```python
from build123d import *

# Parameters (mm, degrees)
SKETCH1_R           = 10
BOSS_EXTRUDE1_DEPTH = 80
FILLET1_R           = 10
BOSS_EXTRUDE2_START = 64
SKETCH2_R           = 12
SKETCH2_R_2         = 10
BOSS_EXTRUDE2_DEPTH = 6


with BuildPart() as part:
    # Sketch1 → Boss-Extrude1 (new body)
    with BuildSketch(Plane.XY):
        Circle(SKETCH1_R)
    extrude(amount=BOSS_EXTRUDE1_DEPTH)

    # Fillet1
    fillet1_edges = [part.edges().sort_by_distance(p)[0] for p in [
        (-10, 0, 80),
    ]]
    fillet(fillet1_edges, radius=FILLET1_R)

    # Sketch2 → Boss-Extrude2 (add)
    with BuildSketch(Plane.XY.offset(BOSS_EXTRUDE2_START)):
        Circle(SKETCH2_R)
        Circle(SKETCH2_R_2, mode=Mode.SUBTRACT)
    extrude(amount=BOSS_EXTRUDE2_DEPTH)


solid = part.part
```
Build history of the part. All positions in model axes, mm. A direction names the side the tool comes from. Give positions to 0.01 mm unless a question says otherwise; leave off trailing zeros. Loops run counter-clockwise (first coordinate to the right, second up) from the corner with the lowest first, then second, coordinate; pieces in that order, holes last.
Item 1: Drill centre lines: line 1 (X direction, y = 0.5, z = 51.5); line 2 (Y direction, x = 0, z = 61); line 3 (Z direction, x = 3.75, y = 10.5). Where is each one in solid material? Low to high.
Answers follow:
line 1: x = -9.99 to 9.99
line 2: y = -10 to 10
line 3: z = 64 to 70
Item 2: Slice it at A-A, the plane x = 0. List the corners of the cut face in (y, z), and give its area (3 significant figures).
Answers follow:
outline: (-12, 64) - (-10, 64) - (-10, 0) - (10, 0) - (10, 64) - (12, 64) - (12, 70) - (10, 70) arc R10 ccw to (-10, 70) - (-12, 70) - close
area: 1,580 mm2
Item 3: Slice it at C-C, the plane z = 43.5. List the corners of the cut face in (x, y).
Answers follow:
outline: circle Ø20 at (0, 0)
Item 4: Flat gauge pins, fed straight in: pin 1 (4 mm diameter, centred on y = 6.5, z = 23.5, fed in from +X); pin 2 (2 mm diameter, centred on x = -6, z = 38.5, fed in from +Y); pin 3 (6 mm diameter, centred on x = -6.5, y = 3, fed in from +Z). Where does each tip first touch, or does it go through?
Answers follow:
pin 1: stops at x = 8.93
pin 2: stops at y = 8.66
pin 3: stops at z = 79.09
Item 5: Which spindle directions (+Z, -Z, +X, -X, +Y, -Y) get a long thin tool onto all of the face, cutting with end or side? Do faces 1 (the face through (-2.17, -9.76, 31.55)), 2 (the face through (0, 0, 0)), 3 (the face through (-5, 9, 70)). Say none if no direction does.
Answers follow:
face 1: -Z
face 2: -Z, +X, -X, +Y, -Y
face 3: +Z
